from build123d import *

# Parameters (mm, degrees)
SKETCH3_W            = 220
SKETCH3_H            = 220
BOSS_EXTRUDE1_DEPTH  = 10
CUT_EXTRUDE1_DEPTH   = 10
SKETCH5_W            = 450
SKETCH5_H            = 450
SKETCH5_W_2          = 400
SKETCH5_H_2          = 400
BOSS_EXTRUDE3_DEPTH  = 25
CUT_EXTRUDE2_DEPTH   = 25
SKETCH9_W            = 450
SKETCH9_H            = 50
CUT_EXTRUDE3_DEPTH   = 25
SKETCH10_W           = 450
SKETCH10_H           = 40
CUT_EXTRUDE4_DEPTH   = 25
SKETCH11_W           = 25
SKETCH11_H           = 25
BOSS_EXTRUDE5_DEPTH  = 25
SKETCH12_W           = 25
SKETCH12_H           = 25
BOSS_EXTRUDE6_DEPTH  = 25
SKETCH13_W           = 25
SKETCH13_H           = 25
BOSS_EXTRUDE7_DEPTH  = 25
SKETCH14_R           = 5
CUT_EXTRUDE5_DEPTH   = 25
BOSS_EXTRUDE8_DEPTH  = 25
BOSS_EXTRUDE9_DEPTH  = 25
CUT_EXTRUDE6_DEPTH   = 25
BOSS_EXTRUDE10_DEPTH = 25
BOSS_EXTRUDE11_DEPTH = 25
BOSS_EXTRUDE12_DEPTH = 400
BOSS_EXTRUDE13_DEPTH = 400
CUT_EXTRUDE7_DEPTH   = 450
SKETCH24_W           = 50
SKETCH24_H           = 59.452998038
CUT_EXTRUDE8_DEPTH   = 350
SKETCH25_W           = 25
SKETCH25_H           = 59.452998038
BOSS_EXTRUDE14_DEPTH = 35
SKETCH26_W           = 12.5
SKETCH26_H           = 172.55
BOSS_EXTRUDE15_DEPTH = 12.5
SKETCH27_W           = 12.5
SKETCH27_H           = 12.5
BOSS_EXTRUDE16_DEPTH = 12.5
SKETCH28_R           = 2.5
CUT_EXTRUDE9_DEPTH   = 12.5
SKETCH29_W           = 116.183817877
SKETCH29_H           = 120.115800598
CUT_EXTRUDE10_DEPTH  = 800


with BuildPart() as part:
    # Sketch3 → Boss-Extrude1 (new body)
    with BuildSketch(Plane(origin=(0, 0, 0), x_dir=(1, 0, 0), z_dir=(0, 1, 0))):
        Rectangle(SKETCH3_W, SKETCH3_H)
    extrude(amount=BOSS_EXTRUDE1_DEPTH)

    # Sketch4 → Cut-Extrude1 (cut)
    with BuildSketch(Plane(origin=(0, 10, 0), x_dir=(1, 0, 0), z_dir=(0, 1, 0))):
        Polygon((0, -110), (-110, 110), (-110, -110), align=None)
        Polygon((110, 110), (0, -110), (110, -110), align=None)
    extrude(amount=-CUT_EXTRUDE1_DEPTH, mode=Mode.SUBTRACT)

    # Sketch17 → Cut-Extrude6 (cut)
    with BuildSketch(Plane(origin=(0, 10, 0), x_dir=(1, 0, 0), z_dir=(0, 1, 0))):
        Polygon((-110, 110), (110, 110), (0, -110), align=None)
    extrude(amount=-CUT_EXTRUDE6_DEPTH, mode=Mode.SUBTRACT)


with BuildPart() as body_2:
    # Sketch5 → Boss-Extrude3 (new body)
    with BuildSketch(Plane.XZ):
        Rectangle(SKETCH5_W, SKETCH5_H)
        Rectangle(SKETCH5_W_2, SKETCH5_H_2, mode=Mode.SUBTRACT)
    extrude(amount=-BOSS_EXTRUDE3_DEPTH)

    # Sketch8 → Cut-Extrude2 (cut)
    with BuildSketch(Plane(origin=(0, 25, 0), x_dir=(1, 0, 0), z_dir=(0, 1, 0))):
        Polygon((-225, 200), (-200, 200), (225, 200), (225, 225), (-225, 225), align=None)
    extrude(amount=-CUT_EXTRUDE2_DEPTH, mode=Mode.SUBTRACT)

    # Sketch9 → Cut-Extrude3 (cut)
    with BuildSketch(Plane(origin=(0, 25, 0), x_dir=(1, 0, 0), z_dir=(0, 1, 0))):
        with Locations((0, 175)):
            Rectangle(SKETCH9_W, SKETCH9_H)
    extrude(amount=-CUT_EXTRUDE3_DEPTH, mode=Mode.SUBTRACT)

    # Sketch10 → Cut-Extrude4 (cut)
    with BuildSketch(Plane(origin=(0, 25, 0), x_dir=(1, 0, 0), z_dir=(0, 1, 0))):
        with Locations((0, 130)):
            Rectangle(SKETCH10_W, SKETCH10_H)
    extrude(amount=-CUT_EXTRUDE4_DEPTH, mode=Mode.SUBTRACT)

    # Sketch11 → Boss-Extrude5 (add)
    with BuildSketch(Plane(origin=(0, 0, -110), x_dir=(-1, 0, 0), z_dir=(0, 0, -1))):
        with Locations((212.5, 12.5)):
            Rectangle(SKETCH11_W, SKETCH11_H)
        with Locations((-212.5, 12.5)):
            Rectangle(SKETCH11_W, SKETCH11_H)
    extrude(amount=BOSS_EXTRUDE5_DEPTH)

    # Sketch12 → Boss-Extrude6 (add)
    with BuildSketch(Plane(origin=(-200, 0, 0), x_dir=(0, 0, -1), z_dir=(1, 0, 0))):
        with Locations((122.5, 12.5)):
            Rectangle(SKETCH12_W, SKETCH12_H)
    extrude(amount=BOSS_EXTRUDE6_DEPTH)

    # Sketch13 → Boss-Extrude7 (add)
    with BuildSketch(Plane.ZY.offset(-200)):
        with Locations((-122.5, 12.5)):
            Rectangle(SKETCH13_W, SKETCH13_H)
    extrude(amount=BOSS_EXTRUDE7_DEPTH)

    # Sketch14 → Cut-Extrude5 (cut)
    with BuildSketch(Plane(origin=(0, 25, 0), x_dir=(1, 0, 0), z_dir=(0, 1, 0))):
        with Locations(Location((-187.5, 122.5, 0), (0, 0, 270))):  # turned: the seam where the file's is
            Circle(SKETCH14_R)
        with Locations(Location((187.5, 122.5, 0), (0, 0, 270))):  # turned: the seam where the file's is
            Circle(SKETCH14_R)
    extrude(amount=-CUT_EXTRUDE5_DEPTH, mode=Mode.SUBTRACT)

    # Sketch15 → Boss-Extrude8 (add)
    with BuildSketch(Plane.ZY.offset(225)):
        Polygon((225, 0), (225, -20), (-135, 0), align=None)
        Polygon((225, 25), (225, 45), (-135, 25), align=None)
    extrude(amount=-BOSS_EXTRUDE8_DEPTH)

    # Sketch16 → Boss-Extrude9 (add)
    with BuildSketch(Plane(origin=(225, 0, 0), x_dir=(0, 0, -1), z_dir=(1, 0, 0))):
        Polygon((-225, 45), (-225, 25), (135, 25), align=None)
        Polygon((-225, 0), (-225, -20), (135, 0), align=None)
    extrude(amount=-BOSS_EXTRUDE9_DEPTH)

    # Sketch18 → Boss-Extrude10 (add)
    with BuildSketch(Plane.ZY.offset(225)):
        Polygon((175.07698234, 42.226499019), (225, 45), (225, 125), align=None)
        Polygon((225, -100), (225, -20), (175.07698234, -17.226499019), align=None)
    extrude(amount=-BOSS_EXTRUDE10_DEPTH)

    # Sketch19 → Boss-Extrude11 (add)
    with BuildSketch(Plane(origin=(225, 0, 0), x_dir=(0, 0, -1), z_dir=(1, 0, 0))):
        Polygon((-225, 125), (-225, 45), (-175.07698234, 42.226499019), align=None)
        Polygon((-225, -20), (-225, -100), (-175.07698234, -17.226499019), align=None)
    extrude(amount=-BOSS_EXTRUDE11_DEPTH)

    # Sketch20 → Boss-Extrude12 (add)
    with BuildSketch(Plane(origin=(-200, 0, 0), x_dir=(0, 0, -1), z_dir=(1, 0, 0))):
        Polygon((-200, 25), (-225, 125), (-225, 25), align=None)
    extrude(amount=BOSS_EXTRUDE12_DEPTH)

    # Sketch21 → Boss-Extrude13 (add)
    with BuildSketch(Plane(origin=(-200, 0, 0), x_dir=(0, 0, -1), z_dir=(1, 0, 0))):
        Polygon((-225, 0), (-225, -100), (-200, 0), align=None)
    extrude(amount=BOSS_EXTRUDE13_DEPTH)

    # Sketch22 → Cut-Extrude7 (cut)
    with BuildSketch(Plane.ZY.offset(225)):
        Polygon((175.07698234, -17.226499019), (175.07698234, 42.226499019), (225, 125), (225, -100), align=None)
    extrude(amount=-CUT_EXTRUDE7_DEPTH, mode=Mode.SUBTRACT)

    # Sketch24 → Cut-Extrude8 (cut)
    with BuildSketch(Plane.XY.offset(175.07698234)):
        with Locations((-200, 12.5)):
            Rectangle(SKETCH24_W, SKETCH24_H)
    extrude(amount=-CUT_EXTRUDE8_DEPTH, mode=Mode.SUBTRACT)

    # Sketch25 → Boss-Extrude14 (add)
    with BuildSketch(Plane.XY.offset(175.07698234)):
        with Locations((212.5, 12.5)):
            Rectangle(SKETCH25_W, SKETCH25_H)
    extrude(amount=BOSS_EXTRUDE14_DEPTH)

    # Sketch29 → Cut-Extrude10 (cut)
    with BuildSketch(Plane.XY.offset(210.07698234)):
        with Locations((211.346821748, 11.078491342)):
            Rectangle(SKETCH29_W, SKETCH29_H)
    extrude(amount=-CUT_EXTRUDE10_DEPTH, mode=Mode.SUBTRACT)


with BuildPart() as body_2_2:
    # Sketch26 → Boss-Extrude15 (new body)
    with BuildSketch(Plane.XZ.offset(17.226499019)):
        Rectangle(SKETCH26_W, SKETCH26_H)
        Polygon((14.85, 86.275), (6.25, 86.275), (6.25, -86.275), (14.85, 68.775), align=None)
        Polygon((-14.85, 68.775), (-14.85, 86.275), (-6.25, 86.275), (-6.25, -86.275), align=None)
    extrude(amount=-BOSS_EXTRUDE15_DEPTH)

    # Sketch27 → Boss-Extrude16 (add)
    with BuildSketch(Plane(origin=(0, -4.726499019, 0), x_dir=(1, 0, 0), z_dir=(0, 1, 0))):
        with Locations((0, 80.025)):
            Rectangle(SKETCH27_W, SKETCH27_H)
    extrude(amount=BOSS_EXTRUDE16_DEPTH)

    # Sketch28 → Cut-Extrude9 (cut)
    with BuildSketch(Plane.ZY.offset(6.25)):
        with Locations((-80.025, 1.523500981)):
            Circle(SKETCH28_R)
    extrude(amount=-CUT_EXTRUDE9_DEPTH, mode=Mode.SUBTRACT)


solid = body_2_2.part
Part model, mm, in its own coordinate system. A direction names the side the tool comes from. Round coordinates to 2 decimals unless told otherwise and drop trailing zeros. Write each loop counter-clockwise with the first axis right and the second up, starting at its lowest first coordinate (ties: lowest second). Pieces come first, ordered by that corner, then holes. Notation, with made-up numbers: (-32.75, 40) - (2.25, 40) arc R11 cw to (2.25, 54) - close; hole circle Ø1 at (71.25, 75). An arc over 180 degrees is marked (long way). Use CSV: the item, a comma, the result in double quotes.
Item 1: Slice it at B-B, the plane x = -3. Write the cut outline in (y, z) (1 decimal).
Results list:
outline,"(-17.2, -86.3) - (7.8, -86.3) - (7.8, -73.8) - (-4.7, -73.8) - (-4.7, 86.3) - (-17.2, 86.3) - close; hole circle Ø5 at (1.5, -80)"
Item 2: Slice it at D-D, the plane x = 8.25. Write the cut outline in (y, z) (1 decimal), then the cut area to 3 significant figures.
Results list:
outline,"(-17.2, -50.2) - (-4.7, -50.2) - (-4.7, 86.3) - (-17.2, 86.3) - close"
area,"1,710 mm²"
Item 3: Wall check: L1, parallel to Y at x = -6, z = 57; L2, parallel to Z at x = 4.25, y = -3.5 (3 decimals); L3, parallel to Z at x = -3, y = 0.5 (3 decimals). Give the ranges that are in metal, low to high.
Results list:
L1,"y = -17.23 to -4.73"
L2,"z = -86.275 to -73.775"
L3,"z = -86.275 to -82.306, -77.744 to -73.775"
Item 4: Slice it at C-C, the plane z = 75.5. Write the cut outline in (x, y).
Results list:
outline,"(-14.85, -17.23) - (14.85, -17.23) - (14.85, -4.73) - (-14.85, -4.73) - close"
Item 5: Slice it at A-A, the plane y = -11.5. Write the cut outline in (x, z) (3 decimals), then the cut area to 3 significant figures.
Results list:
outline,"(-14.85, 68.775) - (-6.25, -86.275) - (6.25, -86.275) - (14.85, 68.775) - (14.85, 86.275) - (-14.85, 86.275) - close"
area,"3,790 mm²"
Item 6: Flat gauge pins, fed straight in: P1, Ø8, axis at x = 7.5, y = -7, coming from the -Z side (3 decimals); P2, Ø4, axis at y = -0.5, z = -81.5, coming from the +X side; P3, Ø4, axis at x = -1.5, y = 0.5, coming from the +Z side (3 decimals); P4, Ø8, axis at y = -7, z = -51.5, coming from the +X side. Where does each tip first touch, or does it go through?
Results list:
P1,"stops at z = -86.275"
P2,"stops at x = 6.25"
P3,"stops at z = -73.775"
P4,"stops at x = 8.4"
Item 7: Tool access for faces 4 (the flat face through (10.49, -11.06, -9.84)), 5 (the flat face through (0, 1, -73.775)), 6 (the flat face through (6.25, 1, -83)), 7 (the flat face through (-6.25, 1, -83)): list every direction of +Z, -Z, +X, -X, +Y, -Y with a clear straight run to the whole face (end or side of a thin tool).
Results list:
face 4,"-Z, +X, +Y, -Y"
face 5,"+Z, +X, -X, +Y"
face 6,"+Z, -Z, +X, +Y"
face 7,"+Z, -Z, -X, +Y"
Item 8: Pull direction Y, two halves, no side cores. Call faces 1 (the flat face through (0, 7.774, -80)), 2 (the flat face through (0, -5, -86.275)), 3 (the cylindrical face through (-0.09, 2.27, -77.64)): pulls with the +Y half, pulls with the -Y half, needs draft (parallel to the pull), parting line crosses it, or undercut.
Results list:
face 1,"pulls with the +Y half"
face 2,"needs draft"
face 3,"undercut"
